from build123d import *


with BuildPart() as part:
    # Sketch1 → Revolve1 (revolve)
    with BuildSketch(Plane.XZ, mode=Mode.PRIVATE) as revolve1_sk:
        with BuildLine():
            Line((25.3, 0), (27.7, 0))
            Line((27.7, 0), (27.7, 1.5))
            Line((27.7, 1.5), (26.5, 1.5))
            Line((26.5, 1.5), (26.5, 4.5))
            Line((26.5, 4.5), (27.7, 4.5))
            Line((27.7, 4.5), (27.7, 6))
            Line((27.7, 6), (26.5, 6))
            Line((26.5, 6), (26.5, 28))
            Line((26.5, 28), (27.7, 28))
            Line((27.7, 28), (27.7, 29.5))
            Line((27.7, 29.5), (26.5, 29.5))
            Line((26.5, 29.5), (26.5, 32.5))
            Line((26.5, 32.5), (27.7, 32.5))
            Line((27.7, 32.5), (27.7, 34))
            Line((27.7, 34), (27.3, 34))
            ThreePointArc((27.3, 34), (25.885786438, 33.414213562), (25.3, 32))
            Line((25.3, 32), (25.3, 0))
        make_face()
    revolve(revolve1_sk.sketch.rotate(Axis((0, 0, 34), (0, 0, -1)), 180), axis=Axis((0, 0, 34), (0, 0, -1)))


solid = part.part
CAD build for the part. Positions are in the model's coordinates, mm. A direction names the side the tool comes from. Coordinates: 2 decimals unless noted, no trailing zeros. Loops run counter-clockwise (first coordinate to the right, second up) from the corner with the lowest first, then second, coordinate; pieces in that order, holes last. Notation, with made-up numbers: (39, 50) -> (83, 50) arc R25 ccw to (83, 73) -> close; hole circle Ø9 at (51.5, 10). An arc over 180 degrees is marked (long way). One line per item, written item: value.
1. Flat gauge pins, fed straight in: P1, Ø6, axis at y = 12, z = 4, coming from the +X side; P2, Ø1.5, axis at x = -14, z = 29, coming from the +Y side; P3, Ø1, axis at x = 6, z = 22.5, coming from the +Y side; P4, Ø16.5, axis at x = -10, y = 8.5, coming from the -Z side. Where does each tip first touch, or does it go through?
Answers:
P1: stops at x = 26.18
P2: stops at y = 24.33
P3: stops at y = 25.92
P4: passes through
2. Slice it at C-C on z = 3.5. Write the cut outline in (x, y).
Answers:
outline: circle Ø53 at (0, 0); hole circle Ø50.6 at (0, 0)
3. Drill centre lines: line 1 (Y direction, x = 0, z = 17); line 2 (X direction, y = -3, z = 30.5); line 3 (X direction, y = -15, z = 19.5). Where is each one in solid material? Low to high. Write a range as [from, to].
Answers:
line 1: y = [-26.5, -25.3], [25.3, 26.5]
line 2: x = [-26.33, -25.12], [25.12, 26.33]
line 3: x = [-21.85, -20.37], [20.37, 21.85]
4. Which spindle directions (+Z, -Z, +X, -X, +Y, -Y) get a long thin tool onto all of the face, cutting with end or side? Do faces 1 (the face through (-2, -27, 29.5)), 2 (the face through (6.005, -27.041, 5.26)). Say none if no direction does.
Answers:
face 1: none
face 2: +Z, -Z
5. Pull direction Z, two halves, no side cores. Call faces 3 (the face through (6.005, -27.041, 33.26)), 4 (the face through (-2, -27, 6)), 5 (the face through (-2, -27, 1.5)), 6 (the face through (12.2, -22.4, 0)): pulls with the +Z half, pulls with the -Z half, needs draft (parallel to the pull), parting line crosses it, or undercut.
Answers:
face 3: needs draft
face 4: undercut
face 5: undercut
face 6: pulls with the -Z half
